Design review of the part shown in the three views and the two pictorial views. Dimensions are in mm from the part's minimum x, y and z. Give positions to 0.01 mm unless a question says otherwise; leave off trailing zeros. Loops run counter-clockwise (first coordinate to the right, second up) from the corner with the lowest first, then second, coordinate; pieces in that order, holes last. Notation, with made-up numbers: (72.25, -18) -> (130.25, -18) arc R25 ccw to (130.25, 14) -> close; hole circle Ø5 at (82, -8.5). An arc over 180 degrees is marked (long way). Answer as CSV lines item,"result".
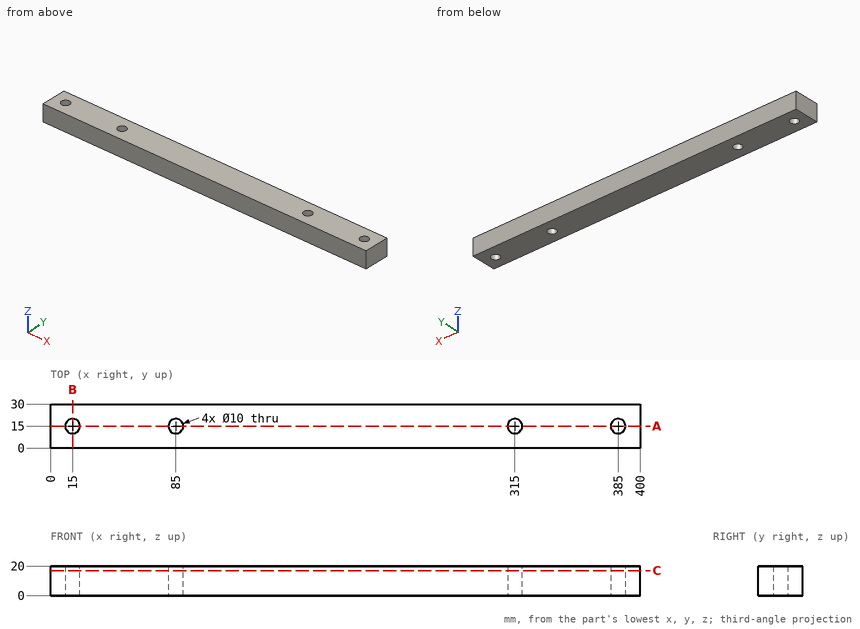
Q1. We need section A-A, the plane y = 15. State the section outline as (x, z) points.
Filled sheet:
outline,"(0, 0) -> (10, 0) -> (10, 20) -> (0, 20) -> close; (20, 0) -> (80, 0) -> (80, 20) -> (20, 20) -> close; (90, 0) -> (310, 0) -> (310, 20) -> (90, 20) -> close; (320, 0) -> (380, 0) -> (380, 20) -> (320, 20) -> close; (390, 0) -> (400, 0) -> (400, 20) -> (390, 20) -> close"
Q2. We need section C-C, the plane z = 17. State the section outline as (x, y) points, and give its area (3 significant figures).
Filled sheet:
outline,"(0, 0) -> (400, 0) -> (400, 30) -> (0, 30) -> close; hole circle Ø10 at (15, 15); hole circle Ø10 at (85, 15); hole circle Ø10 at (315, 15); hole circle Ø10 at (385, 15)"
area,"11,700 mm^2"
Q3. We need section B-B, the plane x = 15. State the section outline as (y, z) points, and give its area (3 significant figures).
Filled sheet:
outline,"(0, 0) -> (10, 0) -> (10, 20) -> (0, 20) -> close; (20, 0) -> (30, 0) -> (30, 20) -> (20, 20) -> close"
area,"400 mm^2"
Q4. To check wall thickness, follow probe 1 along X at (y, z) = (18.75, 15.5); probe 2 along Y at (x, z) = (85, 15.5); probe 3 along Y at (x, z) = (311, 10). State the ranges of each line that lie inside material, in increasing order. Write a range as from..to.
Filled sheet:
probe 1,"x = 0..11.69, 18.31..81.69, 88.31..311.69, 318.31..381.69, 388.31..400"
probe 2,"y = 0..10, 20..30"
probe 3,"y = 0..12, 18..30"
